from build123d import *

# Parameters (mm, degrees)
SKETCH1_W           = 20
SKETCH1_H           = 5
BOSS_EXTRUDE1_DEPTH = 64.175
SKETCH2_R           = 1.75
CUT_EXTRUDE1_DEPTH  = 66.14161976


with BuildPart() as part:
    # Sketch1 → Boss-Extrude1 (new, symmetric)
    with BuildSketch(Plane.XY):
        Rectangle(SKETCH1_W, SKETCH1_H)
    extrude(amount=BOSS_EXTRUDE1_DEPTH, both=True)

    # Sketch2 → Cut-Extrude1 (cut, through all)
    with BuildSketch(Plane(origin=(0, 2.5, 0), x_dir=(1, 0, 0), z_dir=(0, 1, 0))):
        with Locations(Location((-6.25, -61, 0), (0, 0, 270))):
            Circle(SKETCH2_R)
        with Locations(Location((6.25, -61, 0), (0, 0, 90))):
            Circle(SKETCH2_R)
        with Locations(Location((6.25, 61, 0), (0, 0, 270))):
            Circle(SKETCH2_R)
        with Locations(Location((-6.25, 61, 0), (0, 0, 90))):
            Circle(SKETCH2_R)
    extrude(amount=-CUT_EXTRUDE1_DEPTH, mode=Mode.SUBTRACT)


solid = part.part
Source: CAD feature listing. Evaluate the final solid. Frame: model axes, mm. Round coordinates to 2 decimals unless told otherwise and drop trailing zeros. Loops run counter-clockwise (first coordinate to the right, second up) from the corner with the lowest first, then second, coordinate; pieces in that order, holes last.
Q1. Section A-A, the plane x = -6.25. Return loops of the section in (y, z) (3 decimals), plus the area to 3 significant figures.
Q2. Section B-B, the plane z = -61. Return loops of the section in (x, y).
Q3. Mould query, pull axis X, two halves, no side actions, for faces 1 (the face through (0, 0, 64.175)), 2 (the face through (-10, 0, 1)), 3 (the face through (-6.92, 0.035, 62.617)). Classes: pulls with the +X half, pulls with the -X half, needs draft (parallel to the pull), parting line crosses it, or undercut.
Q4. Ray query, line 1 (Z direction, x = -6.5, y = 0.6) (3 decimals); line 2 (X direction, y = 0.75, z = -61); line 3 (Z direction, x = -7, y = -0.25) (3 decimals). Return the intervals inside material, ascending.
Q5. First-contact query: P1, Ø3, axis at x = 6.25, z = 61, coming from the +Y side. Flat tip, straight axial feed; report the tip coordinate or a pass-through.
Solutions:
1. outline: (-2.5, -64.175) - (2.5, -64.175) - (2.5, -62.75) - (-2.5, -62.75) - close; (-2.5, -59.25) - (2.5, -59.25) - (2.5, 59.25) - (-2.5, 59.25) - close; (-2.5, 62.75) - (2.5, 62.75) - (2.5, 64.175) - (-2.5, 64.175) - close
1. area: 607 mm2
2. outline: (-10, -2.5) - (-8, -2.5) - (-8, 2.5) - (-10, 2.5) - close; (-4.5, -2.5) - (4.5, -2.5) - (4.5, 2.5) - (-4.5, 2.5) - close; (8, -2.5) - (10, -2.5) - (10, 2.5) - (8, 2.5) - close
3. face 1: needs draft
3. face 2: pulls with the -X half
3. face 3: undercut
4. line 1: z = -64.175 to -62.732, -59.268 to 59.268, 62.732 to 64.175
4. line 2: x = -10 to -8, -4.5 to 4.5, 8 to 10
4. line 3: z = -64.175 to -62.581, -59.419 to 59.419, 62.581 to 64.175
5. P1: passes through
